from build123d import *

# Parameters (mm, degrees)
SKETCH1_W           = 10
SKETCH1_H           = 30
BOSS_EXTRUDE1_DEPTH = 2
SKETCH2_W           = 10
SKETCH2_H           = 31.258977403
BOSS_EXTRUDE2_DEPTH = 2
BOSS_EXTRUDE3_DEPTH = 10


with BuildPart() as part:
    # Sketch1 → Boss-Extrude1 (new body)
    with BuildSketch(Plane.XY):
        with Locations((-0.545023697, 5.355450237)):
            Rectangle(SKETCH1_W, SKETCH1_H)
    extrude(amount=BOSS_EXTRUDE1_DEPTH)

    # Sketch2 → Boss-Extrude2 (add)
    with BuildSketch(Plane(origin=(0, -1.262673113, 4.403464453), x_dir=(1, 0, 0), z_dir=(0, -0.275637356, 0.961261696))):
        with Locations((-0.545023697, 6.909827152)):
            Rectangle(SKETCH2_W, SKETCH2_H)
    extrude(amount=-BOSS_EXTRUDE2_DEPTH)

    # Sketch3 → Boss-Extrude3 (add)
    with BuildSketch(Plane.ZY.offset(5.545023697)):
        with BuildLine():
            Line((2, 6.250675975), (2, -2.388639206))
            Line((2, -2.388639206), (4.496805616, 6.318756763))
            add(Edge.make_bspline(
                [(2, 6.250675975), (2.210821092, 5.681941721), (3.390467427, 4.618454358), (4.496805616, 6.318756763)],
                knots=[0, 0, 0, 0, 1, 1, 1, 1], degree=3))
        make_face()
    extrude(amount=-BOSS_EXTRUDE3_DEPTH)


solid = part.part
Geometry: final body of the model. Coordinates: model frame, mm. A direction names the side the tool comes from. Coordinates: 2 decimals unless noted, no trailing zeros. Order: outer loops, then holes, each group sorted by start corner. A loop starts at its lowest first (then second) coordinate and runs counter-clockwise, first axis right, second up.
(1) Section query B-B (z = 1). Return the cut outline in (x, y), plus the area to 3 significant figures.
(2) Access query for faces 1 (the face through (-1, 6, 0)), 2 (the face through (-1, 20.355, 1)). Directions: +Z, -Z, +X, -X, +Y, -Y. A direction counts if a zero-diameter tool reaches every point of the face in a straight line with its end or side. Return the directions, or none.
(3) Section query C-C (y = -4.5). Return the cut outline in (x, z).
(4) Material intervals for probe 1 along Y at (x, z) = (-4.5, 1.5); probe 2 along Z at (x, y) = (2.25, 18); probe 3 along Z at (x, y) = (1, 17), sorted ascending.
(5) Section query A-A (y = 17.5). Return the cut outline in (x, z), plus the area to 3 significant figures.
(6) First-contact query: pin 1 (0.6 mm diameter, centred on x = -0.5, z = 0.5, fed in from +Y); pin 2 (3 mm diameter, centred on x = -3, z = 7.5, fed in from +Y). Flat tips, straight axial feed; report the tip coordinate or a pass-through.
(7) Draft query along Z for faces 3 (the face through (-1, 13, 2)), 4 (the face through (-0.62, 5.59, 6.37)), 5 (the face through (-5.545, 5.9, 1.7)), 6 (the face through (-0.615, 13.739, 6.625)). Return one class per face: pulls with the +Z half, pulls with the -Z half, needs draft (parallel to the pull), parting line crosses it, or undercut.
Solution:
1. outline: (-5.55, -9.64) - (4.45, -9.64) - (4.45, 20.36) - (-5.55, 20.36) - close
1. area: 300 mm2
2. face 1: -Z, +X, -X, +Y, -Y
2. face 2: -Z, +X, -X, +Y
3. outline: (-5.55, 0) - (4.45, 0) - (4.45, 3.48) - (-5.55, 3.48) - close
4. probe 1: y = -9.64 to 20.36
4. probe 2: z = 0 to 2, 7.85 to 9.93
4. probe 3: z = 0 to 2, 7.56 to 9.64
5. outline: (-5.55, 0) - (4.45, 0) - (4.45, 2) - (-5.55, 2) - close; (-5.55, 7.7) - (4.45, 7.7) - (4.45, 9.78) - (-5.55, 9.78) - close
5. area: 40.8 mm2
6. pin 1: stops at y = 20.36
6. pin 2: stops at y = 20.95
7. face 3: undercut
7. face 4: pulls with the +Z half
7. face 5: needs draft
7. face 6: undercut
